Answer from the drawing. Dimensions are ordinates in mm from the lowest x, y and z of the part. A direction names the side the tool comes from. Give positions to 0.01 mm unless a question says otherwise; leave off trailing zeros. Write each loop counter-clockwise with the first axis right and the second up, starting at its lowest first coordinate (ties: lowest second). Pieces come first, ordered by that corner, then holes. Notation, with made-up numbers: M 68.25,81 L 87.25,81 A7 cw 87.25,91 Z; hole C 47.5,85.5 d1. An arc over 180 degrees is marked long. Answer as a JSON object with one key per item and string values.
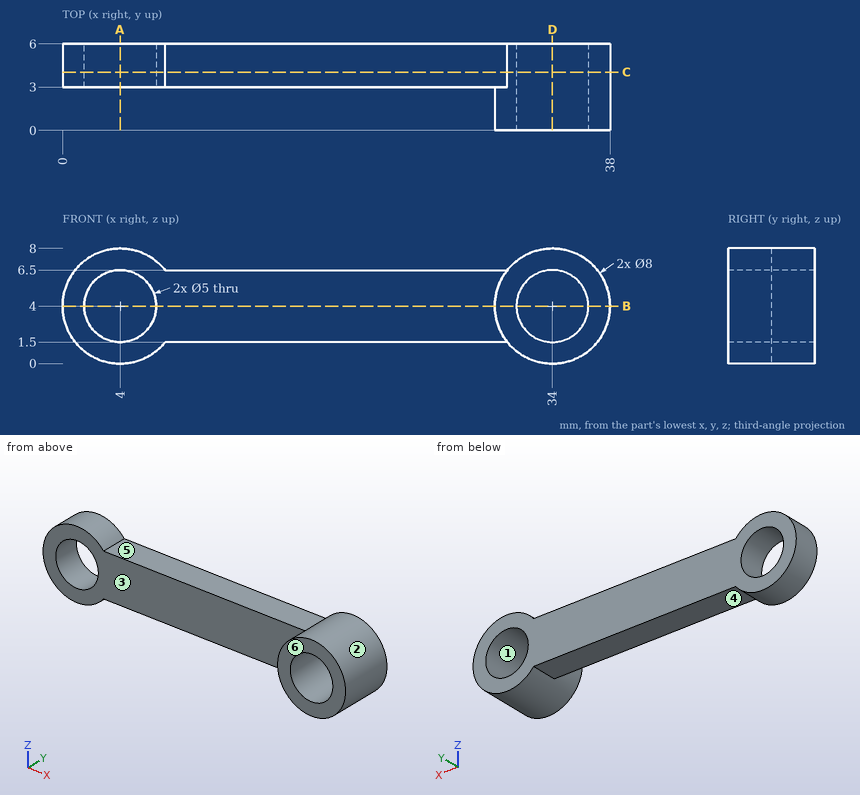
1. For the marked faces 4, 5 and 6, determine the directions among +Z, -Z, +X, -X, +Y, -Y from which every point of the face is accessible in a straight line to the end or side of a thin tool.
Verdict:
{"face 4": "-Z, +Y, -Y", "face 5": "+Z, +Y, -Y", "face 6": "+Z, -Z, +X, -X, -Y"}
2. A cutting plane is placed at D-D, the plane x = 34. Give the vertices of the cut face in (y, z).
Verdict:
{"outline": "M 0,0 L 6,0 L 6,1.5 L 0,1.5 Z; M 0,6.5 L 6,6.5 L 6,8 L 0,8 Z"}
3. The mould has two halves that part along Z. Classify the marked faces 1, 2 and 3: released by +Z, released by -Z, zero draft, split by the parting line, or undercut.
Verdict:
{"face 1": "undercut", "face 2": "split by the parting line", "face 3": "zero draft"}
4. A cutting plane is placed at B-B, the plane z = 4. Give the vertices of the cut face in (x, y).
Verdict:
{"outline": "M 0,3 L 1.5,3 L 1.5,6 L 0,6 Z; M 6.5,3 L 30,3 L 30,0 L 31.5,0 L 31.5,6 L 6.5,6 Z; M 36.5,0 L 38,0 L 38,6 L 36.5,6 Z"}
5. Consider line 1 along X through (y, z) = (5.05, 4); line 2 along Z through (x, y) = (34, 2.75); line 3 along X through (y, z) = (3.3, 6). Determine where each line is inside the solid, lowest interval first.
Verdict:
{"line 1": "x = 0 to 1.5, 6.5 to 31.5, 36.5 to 38", "line 2": "z = 0 to 1.5, 6.5 to 8", "line 3": "x = 0.54 to 2.5, 5.5 to 32.5, 35.5 to 37.46"}
6. Flat-ended cylindrical pins translate along their axes: pin 1 (4 mm diameter, centred on x = 15, z = 3.5, fed in from -Y); pin 2 (3.5 mm diameter, centred on x = 18, y = 4, fed in from -Z); pin 3 (4 mm diameter, centred on x = 32.5, z = 6, fed in from -Y); pin 4 (0.9 mm diameter, centred on x = 21.5, y = 5, fed in from +Z). Find the tip coordinate at first contact, or state that the pin passes through.
Verdict:
{"pin 1": "stops at y = 3", "pin 2": "stops at z = 1.5", "pin 3": "stops at y = 0", "pin 4": "stops at z = 6.5"}
7. A cutting plane is placed at A-A, the plane x = 4. Give the vertices of the cut face in (y, z), plus the area to 3 significant figures.
Verdict:
{"outline": "M 3,0 L 6,0 L 6,1.5 L 3,1.5 Z; M 3,6.5 L 6,6.5 L 6,8 L 3,8 Z", "area": "9.00 mm2"}
8. A cutting plane is placed at C-C, the plane y = 4.05. Give the vertices of the cut face in (x, z).
Verdict:
{"outline": "M 7.12,1.5 L 30.88,1.5 A4 ccw long 30.88,6.5 L 7.12,6.5 A4 ccw long Z; hole C 4,4 d5; hole C 34,4 d5"}
